Source: three-view drawing plus pictorial views. Frame: mm from the lowest corner of the part. A direction names the side the tool comes from. Give positions to 0.01 mm unless a question says otherwise; leave off trailing zeros. Write each loop counter-clockwise with the first axis right and the second up, starting at its lowest first coordinate (ties: lowest second). Pieces come first, ordered by that corner, then holes. Notation, with made-up numbers: (42, 4.5) -> (47, 4.5) arc R7 ccw to (47, 12.5) -> close; hole circle Ø4 at (16, -17.5). An arc over 180 degrees is marked (long way). Write item = value, one per line.
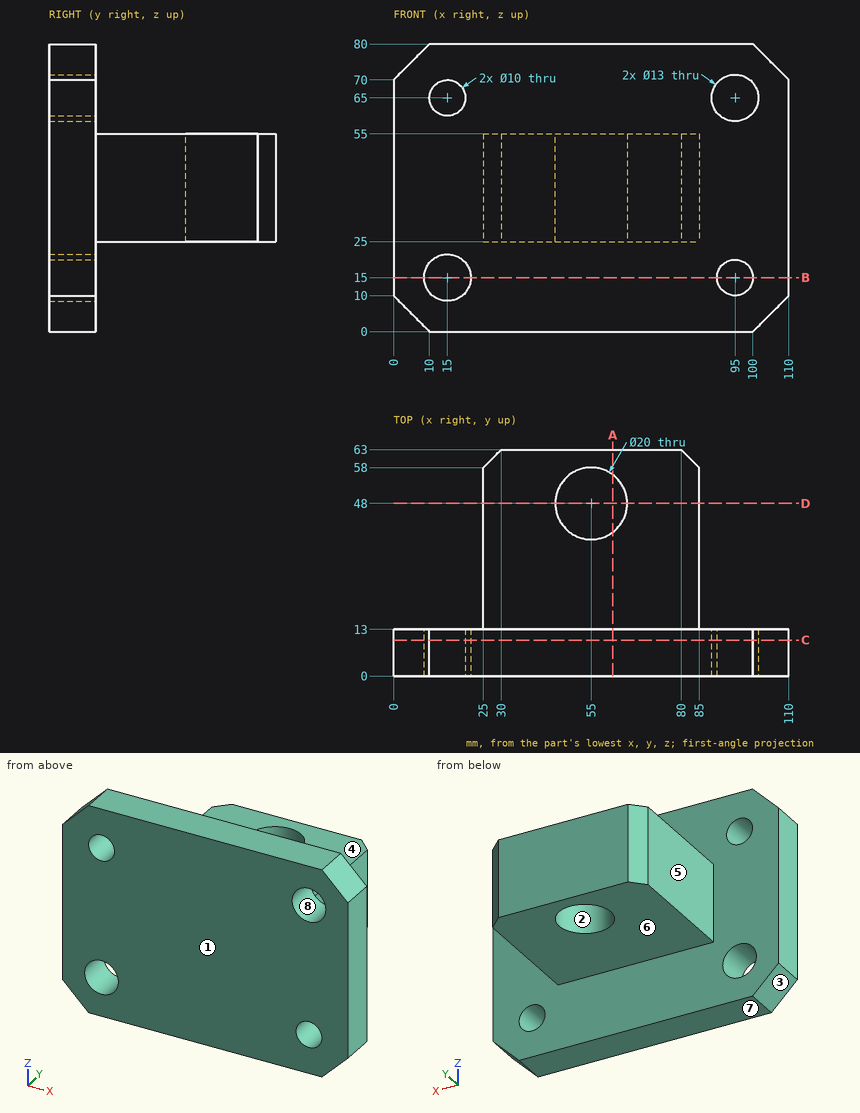
1) Contact query for flat-ended pins moving along their axis: pin 1 (1 mm diameter, centred on x = 70.5, y = 11.5, fed in from -Z); pin 2 (25 mm diameter, centred on x = 62.5, y = 48.5, fed in from +Z); pin 3 (15 mm diameter, centred on x = 15, z = 15, fed in from +Y); pin 4 (12 mm diameter, centred on x = 55, y = 48, fed in from +Z). Output: stop coordinate, or through.
Computed:
pin_1 = 0
pin_2 = 55
pin_3 = 13
pin_4 = through
2) Material intervals for L1, parallel to X at y = 8.25, z = 65; L2, parallel to X at y = 3, z = 15; L3, parallel to Z at x = 95, y = 8, sorted ascending.
Computed:
L1 = 0 to 10, 20 to 88.5, 101.5 to 110
L2 = 0 to 8.5, 21.5 to 90, 100 to 110
L3 = 0 to 10, 20 to 58.5, 71.5 to 80
3) Cut plane A-A (x = 61). Return the cut outline in (y, z), then the cut area to 3 significant figures.
Computed:
outline = (0, 0) -> (13, 0) -> (13, 25) -> (40, 25) -> (40, 55) -> (13, 55) -> (13, 80) -> (0, 80) -> close; (56, 25) -> (63, 25) -> (63, 55) -> (56, 55) -> close
area = 2,060 mm²
4) Cut plane D-D (y = 48). Return the cut outline in (x, z), then the cut area to 3 significant figures.
Computed:
outline = (25, 25) -> (45, 25) -> (45, 55) -> (25, 55) -> close; (65, 25) -> (85, 25) -> (85, 55) -> (65, 55) -> close
area = 1,200 mm²
5) Cut plane B-B (z = 15). Return the cut outline in (x, y).
Computed:
outline = (0, 0) -> (8.5, 0) -> (8.5, 13) -> (0, 13) -> close; (21.5, 0) -> (90, 0) -> (90, 13) -> (21.5, 13) -> close; (100, 0) -> (110, 0) -> (110, 13) -> (100, 13) -> close
6) Access query for the marked faces 4, 5, 6, 7 and 8. Directions: +Z, -Z, +X, -X, +Y, -Y. A direction counts if a zero-diameter tool reaches every point of the face in a straight line with its end or side. Return the directions, or none.
Computed:
face_4 = +Z, +X, -X, +Y
face_5 = +Z, -Z, -X, +Y
face_6 = -Z, +X, -X, +Y
face_7 = -Z, +X, -X, +Y, -Y
face_8 = +Y, -Y
7) Cut plane C-C (y = 10). Return the cut outline in (x, z).
Computed:
outline = (0, 10) -> (10, 0) -> (100, 0) -> (110, 10) -> (110, 70) -> (100, 80) -> (10, 80) -> (0, 70) -> close; hole circle Ø13 at (15, 15); hole circle Ø10 at (15, 65); hole circle Ø13 at (95, 65); hole circle Ø10 at (95, 15)
8) Draft query along Y for the marked faces 1, 2 and 3. Return one class per face: pulls with the +Y half, pulls with the -Y half, needs draft (parallel to the pull), parting line crosses it, or undercut.
Computed:
face_1 = pulls with the -Y half
face_2 = undercut
face_3 = needs draft
